Autodesk Inventor part; units mm, degrees
ref_plane "YZ Plane" through (0, 0, 0) normal (1, 0, 0) x (0, 1, 0)
ref_plane "XZ Plane" through (0, 0, 0) normal (0, 1, 0) x (-1, 0, 0)
ref_plane "XY Plane" through (0, 0, 0) normal (0, 0, 1) x (1, 0, 0)
sketch "Sketch1" plane through (0, 0, 0) normal (0, 0, 1) x (1, 0, 0)
  line L0 (-4.1, -22.5) -> (-4.1, -18)
  line L1 (-4.6, -18) -> (-6.8, -18)
  line L2 (-6.8, -18) -> (-6.8, -9.5)
  line L3 (-6.8, -9.5) -> (-4.5, -7.2)
  line L4 (-4.5, -7.2) -> (4.5, -7.2)
  line L5 (4.5, -7.2) -> (6.8, -9.5)
  line L6 (6.8, -9.5) -> (6.8, -18)
  line L7 (4.1, -18) -> (4.1, -22.5)
  line L8 (22.5, -4.1) -> (18, -4.1)
  line L9 (18, -4.6) -> (18, -6.8)
  line L10 (18, -6.8) -> (9.5, -6.8)
  line L11 (9.5, -6.8) -> (7.2, -4.5)
  line L12 (7.2, -4.5) -> (7.2, 4.5)
  line L13 (7.2, 4.5) -> (9.5, 6.8)
  line L14 (9.5, 6.8) -> (18, 6.8)
  line L15 (18, 4.1) -> (22.5, 4.1)
  line L16 (22.5, 22.5) -> (22.5, 4.4)
  line L17 (4.1, 22.5) -> (4.1, 18)
  line L18 (4.6, 18) -> (6.8, 18)
  line L19 (6.8, 18) -> (6.8, 9.5)
  line L20 (6.8, 9.5) -> (4.5, 7.2)
  line L21 (4.5, 7.2) -> (-4.5, 7.2)
  line L22 (-4.5, 7.2) -> (-6.8, 9.5)
  line L23 (-6.8, 9.5) -> (-6.8, 18)
  line L24 (-4.1, 18) -> (-4.1, 22.5)
  line L25 (-22.5, 22.5) -> (-4.4, 22.5)
  line L26 (-22.5, 4.1) -> (-18, 4.1)
  line L27 (-18, 6.8) -> (-9.5, 6.8)
  line L28 (-9.5, 6.8) -> (-7.2, 4.5)
  line L29 (-7.2, 4.5) -> (-7.2, -4.5)
  line L30 (-7.2, -4.5) -> (-9.5, -6.8)
  line L31 (-9.5, -6.8) -> (-18, -6.8)
  line L32 (-18, -6.8) -> (-18, -4.6)
  line L33 (-18, -4.1) -> (-22.5, -4.1)
  line L34 (-22.5, -22.5) -> (-22.5, -4.4)
  line L35 (-4.4, -22.5) -> (-22.5, -22.5)
  line L36 (-4.5962, -3.182) -> (-3.2627, -1.8485)
  line L37 (-3.2627, 1.8485) -> (-4.5962, 3.182)
  line L38 (-4.5962, 3.182) -> (-3.182, 4.5962)
  line L39 (-3.182, 4.5962) -> (-1.8485, 3.2627)
  line L40 (1.8485, 3.2627) -> (3.182, 4.5962)
  line L41 (3.182, 4.5962) -> (4.5962, 3.182)
  line L42 (4.5962, 3.182) -> (3.2627, 1.8485)
  arc A0 (3.3625, -1.6602) -> (3.3625, 1.6602) centre (0, 0) ccw
  line L43 (3.2627, -1.8485) -> (4.5962, -3.182)
  line L44 (4.5962, -3.182) -> (3.182, -4.5962)
  line L45 (3.182, -4.5962) -> (1.8485, -3.2627)
  line L46 (-1.8485, -3.2627) -> (-3.182, -4.5962)
  line L47 (-3.182, -4.5962) -> (-4.5962, -3.182)
  arc A1 (13.8, -8.8) -> (8.8, -13.8) centre (13.8, -13.8) ccw
  line L48 (13.8, -8.8) -> (20.5, -8.8)
  line L49 (20.5, -8.8) -> (20.5, -15.5)
  arc A2 (15.5, -20.5) -> (20.5, -15.5) centre (15.5, -15.5) ccw
  line L50 (15.5, -20.5) -> (8.8, -20.5)
  line L51 (8.8, -20.5) -> (8.8, -13.8)
  arc A3 (8.8, 13.8) -> (13.8, 8.8) centre (13.8, 13.8) ccw
  line L52 (8.8, 13.8) -> (8.8, 20.5)
  line L53 (8.8, 20.5) -> (15.5, 20.5)
  arc A4 (20.5, 15.5) -> (15.5, 20.5) centre (15.5, 15.5) ccw
  line L54 (20.5, 15.5) -> (20.5, 8.8)
  line L55 (20.5, 8.8) -> (13.8, 8.8)
  arc A5 (-13.8, 8.8) -> (-8.8, 13.8) centre (-13.8, 13.8) ccw
  line L56 (-13.8, 8.8) -> (-20.5, 8.8)
  line L57 (-20.5, 8.8) -> (-20.5, 15.5)
  arc A6 (-15.5, 20.5) -> (-20.5, 15.5) centre (-15.5, 15.5) ccw
  line L58 (-15.5, 20.5) -> (-8.8, 20.5)
  line L59 (-8.8, 20.5) -> (-8.8, 13.8)
  arc A7 (-8.8, -13.8) -> (-13.8, -8.8) centre (-13.8, -13.8) ccw
  line L60 (-8.8, -13.8) -> (-8.8, -20.5)
  line L61 (-8.8, -20.5) -> (-15.5, -20.5)
  arc A8 (-20.5, -15.5) -> (-15.5, -20.5) centre (-15.5, -15.5) ccw
  line L62 (-20.5, -15.5) -> (-20.5, -8.8)
  line L63 (-20.5, -8.8) -> (-13.8, -8.8)
  line L64 (-6.8, 18) -> (-4.1, 18)
  line L65 (4.1, 18) -> (4.6, 18)
  line L66 (-4.4, 22.5) -> (-4.1, 22.5)
  line L67 (4.1, 22.5) -> (22.5, 22.5)
  arc A9 (3.3625, 1.6602) -> (3.2627, 1.8485) centre (0, 0) ccw
  arc A10 (1.8485, 3.2627) -> (-1.6602, 3.3625) centre (0, 0) ccw
  arc A11 (-1.6602, 3.3625) -> (-1.8485, 3.2627) centre (0, 0) ccw
  arc A12 (-3.2627, 1.8485) -> (-3.2627, -1.8485) centre (0, 0) ccw
  arc A13 (-1.8485, -3.2627) -> (-1.6602, -3.3625) centre (0, 0) ccw
  arc A14 (-1.6602, -3.3625) -> (1.8485, -3.2627) centre (0, 0) ccw
  arc A15 (3.2627, -1.8485) -> (3.3625, -1.6602) centre (0, 0) ccw
  line L68 (18, 6.8) -> (18, 4.1)
  line L69 (18, -4.1) -> (18, -4.6)
  line L70 (22.5, 4.4) -> (22.5, 4.1)
  line L71 (22.5, -4.1) -> (22.5, -22.5)
  line L72 (6.8, -18) -> (4.1, -18)
  line L73 (-4.1, -18) -> (-4.6, -18)
  line L74 (22.5, -22.5) -> (4.1, -22.5)
  line L75 (-4.1, -22.5) -> (-4.4, -22.5)
  line L76 (-22.5, -4.4) -> (-22.5, -4.1)
  line L77 (-22.5, 4.1) -> (-22.5, 22.5)
  line L78 (-18, -4.6) -> (-18, -4.1)
  line L79 (-18, 4.1) -> (-18, 6.8)
extrude "Extrusion1" add sketch "Sketch1" along normal blind 2484
ref_plane "Work Plane1" through (0, 0, 1242) normal (0, 0, -1) x (-1, 0, 0)
sketch "Sketch5" plane through (-22.5, 22.5, 2484) normal (0, 1, 0) x (1, 0, 0)
  line L0 (45, 2484) -> (45, 0)
  line L1 (45, 0) -> (26.6, 0)
  circle A0 centre (38.3401, 16) radius 4
  point P0 (22.5, 2484)
  dimension "d19" = 8
  dimension "d20" = 16
extrude "Extrusion5" cut sketch "Sketch5" against normal up to next
mirror "Mirror4" about plane through (0, 0, 1242) normal (0, 0, -1) of "Extrusion5"
properties part number "20.1033.0" material "Aluminum-6061"
Source: CAD feature listing. Evaluate the final solid. Frame: model axes, mm. Coordinates: 2 decimals unless noted, no trailing zeros. One line per item, written item: value. Start each with the question number.
Q1. Contact query for flat-ended pins moving along their axis: P1, Ø1.5, axis at x = -3, z = 1451, coming from the +Y side; P2, Ø5, axis at x = 15.84, z = 2468, coming from the +Y side. Output: stop coordinate, or through.
Q2. Line query: line 1 along X through (y, z) = (14.5, 642); line 2 along X through (y, z) = (19.65, 2468). Output: solid intervals per line, ascending.
Q3. Section query A-A, the plane z = 1812. Give the number of separate pieces and of enclosed holes in the cut face, and give its area (3 significant figures).
Results:
1. P1: y = 7.2
1. P2: y = 8.82
2. line 1: -22.5 to -20.5, -8.8 to -6.8, 6.8 to 8.8, 20.5 to 22.5
2. line 2: -22.5 to -18.29, -8.8 to -4.1, 4.1 to 8.8, 19.84 to 22.5
3. separate pieces: 1
3. enclosed holes: 5
3. area: 748 mm^2
